Verification items for this drawing (mm, ordinates from the low corner). Round coordinates to 2 decimals unless told otherwise and drop trailing zeros. Loops run counter-clockwise (first coordinate to the right, second up) from the corner with the lowest first, then second, coordinate; pieces in that order, holes last. Notation, with made-up numbers: (39.5, -35) - (50.5, -35) arc R26 cw to (50.5, -4) - close; hole circle Ø5 at (3.5, 80.5). An arc over 180 degrees is marked (long way). Put each result on its own line as item: value.
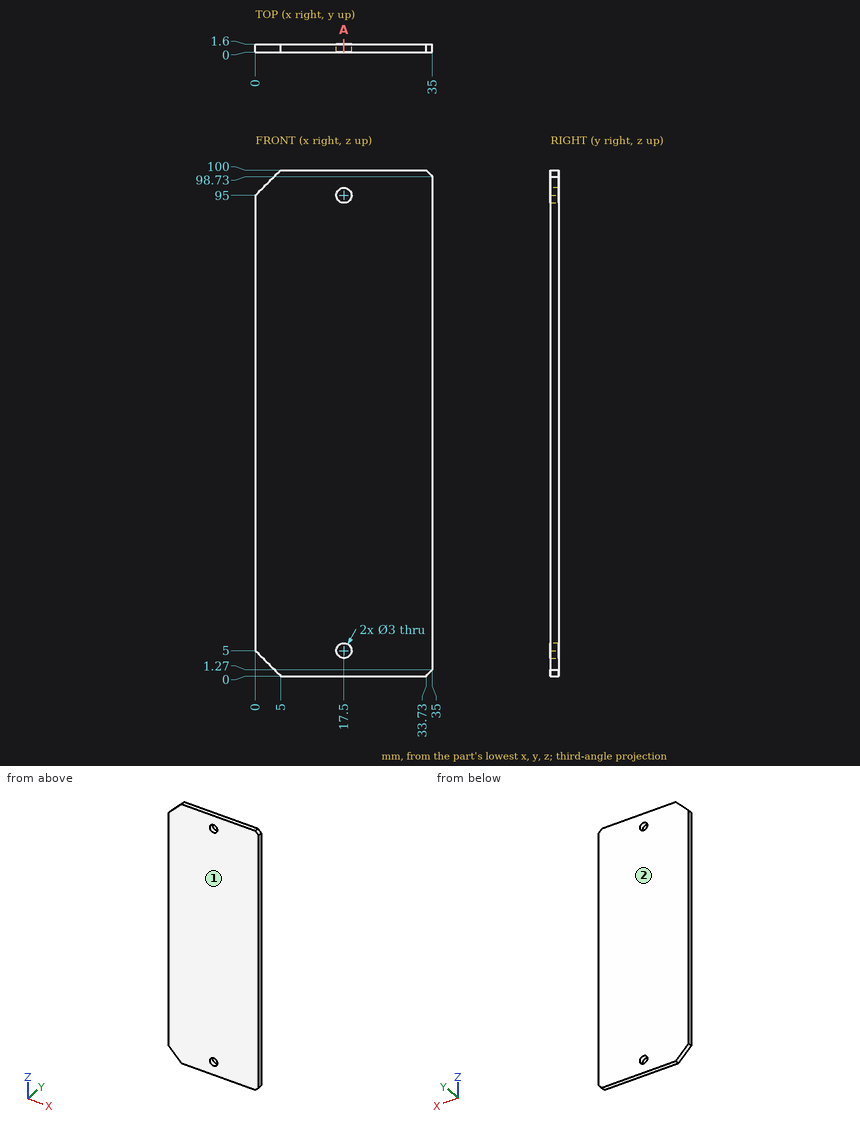
Item 1: Section check A-A on x = 17.5. Enter the section's corners in (y, z).
Filled sheet:
outline: (0, 0) - (1.6, 0) - (1.6, 3.5) - (0, 3.5) - close; (0, 6.5) - (1.6, 6.5) - (1.6, 93.5) - (0, 93.5) - close; (0, 96.5) - (1.6, 96.5) - (1.6, 100) - (0, 100) - close
Item 2: Release check for a two-part mould opening along Y. For the marked faces 1 and 2 record: +Y half, -Y half, draft (parallel to the pull), parting line (faces both ways), or undercut.
Filled sheet:
face 1: -Y half
face 2: +Y half
Item 3: Thickness scan on line 1 (X direction, y = 0.65, z = 5); line 2 (X direction, y = 0.65, z = 4). Record the ranges inside material, lowest first. Write a range as from..to.
Filled sheet:
line 1: 0..16, 19..35
line 2: 1..16.38, 18.62..35
